from build123d import *

# Parameters (mm, degrees)
F0_W       = 355.6
F0_H       = 330.2
F0_R       = 12.7
F1_DEPTH   = 406.4
F2_DEPTH   = 73.81875
F3_SIZE    = 76.2
F4_SIZE2   = 55.4690637022
F4_SIZE    = 152.4
F4_2_SIZE2 = 55.4690637022
F4_2_SIZE  = 152.4
F5_SIZE    = 25.4
F6_SIZE2   = 76.2
F6_SIZE    = 27.7345318511


with BuildPart() as f1:
    # F0 (on Front) → F1 (new body)
    with BuildSketch(Plane.XZ):
        with Locations((-25.4, 165.1)):
            Rectangle(F0_W, F0_H)
        with Locations((-25.4, 127)):
            Circle(F0_R, mode=Mode.SUBTRACT)
        with Locations((-25.4, 127)):
            Circle(F0_R)
    extrude(amount=-F1_DEPTH)

    # F0 (on Front) → F2 (join)
    with BuildSketch(Plane.XZ):
        with Locations((-25.4, 127)):
            Circle(F0_R)
    extrude(amount=F2_DEPTH)

    # F3
    f3_edges = [f1.edges().sort_by_distance(p)[0] for p in [
        (-203.2, 203.2, 330.2),
        (152.4, 203.2, 330.2),
    ]]
    chamfer(f3_edges, length=F3_SIZE)

    # F4
    f4_edges = [f1.edges().sort_by_distance(p)[0] for p in [
        (-203.2, 203.2, 0),
    ]]
    f4_side = f1.faces().sort_by_distance((-203.2, 203.2, 127))[0]
    chamfer(f4_edges, length=F4_SIZE, length2=F4_SIZE2, reference=f4_side)

    # F4#2
    f4_2_edges = [f1.edges().sort_by_distance(p)[0] for p in [
        (152.4, 203.2, 0),
    ]]
    f4_2_side = f1.faces().sort_by_distance((152.4, 203.2, 127))[0]
    chamfer(f4_2_edges, length=F4_2_SIZE, length2=F4_2_SIZE2, reference=f4_2_side)

    # F5
    f5_edges = [f1.edges().sort_by_distance(p)[0] for p in [
        (-165.1, 0, 292.1),
        (-203.2, 0, 203.2),
        (-175.465468, 0, 76.2),
        (-25.4, 0, 0),
        (124.665468, 0, 76.2),
        (152.4, 0, 203.2),
        (114.3, 0, 292.1),
        (-25.4, 0, 330.2),
    ]]
    chamfer(f5_edges, length=F5_SIZE)

    # F6
    f6_edges = [f1.edges().sort_by_distance(p)[0] for p in [
        (-175.465468, 406.4, 76.2),
        (-203.2, 406.4, 203.2),
        (-165.1, 406.4, 292.1),
        (-25.4, 406.4, 330.2),
        (-25.4, 406.4, 0),
        (124.665468, 406.4, 76.2),
        (152.4, 406.4, 203.2),
        (114.3, 406.4, 292.1),
    ]]
    chamfer(f6_edges, length=F6_SIZE, length2=F6_SIZE2)


solid = f1.part
Check sheet for the modelled part. Datum: model origin and axes. Units: mm. A direction names the side the tool comes from. Round coordinates to 2 decimals unless told otherwise and drop trailing zeros. Loops run counter-clockwise (first coordinate to the right, second up) from the corner with the lowest first, then second, coordinate; pieces in that order, holes last. Notation, with made-up numbers: (57.25, 15.25) - (68.25, 15.25) arc R7 ccw to (68.25, 25.25) - close; hole circle Ø11 at (53, 43). An arc over 180 degrees is marked (long way). Answer as CSV lines item,"result". Start each with the question number.
Item 1: Depth check by flat-ended pin: P1, Ø8, axis at y = 4, z = 261.5, coming from the +X side; P2, Ø2, axis at y = 46, z = 96.5, coming from the -X side; P3, Ø2, axis at y = 128.5, z = 98, coming from the +X side. Enter the tip coordinate at first touch or a pass-through.
Item 2: Release check for a two-part mould opening along Y. For faces 1 (the flat face through (113.29, 12.88, 81.55)), 2 (the flat face through (124.277, 199.56, 75.133)), 3 (the flat face through (-26.822, 392.727, 291.567)) record: +Y half, -Y half, draft (parallel to the pull), parting line (faces both ways), or undercut.
Item 3: Section check A-A (x = 10). Record the boundary of the cut face in (y, z), and give its area (3 significant figures).
Item 4: Section check C-C (z = 127). Record the boundary of the cut face in (x, y), and give its area (3 significant figures).
Item 5: Scan lines: line 1 (Y direction, x = 16, z = 156); line 2 (Z direction, x = -137, y = 361.5); line 3 (Y direction, x = -123.5, z = 155.5). Record each from-to range of solid material in increasing order. Write a range as [from, to].
Item 6: Section check B-B (y = 89). Record the boundary of the cut face in (x, z), and give its area (3 significant figures).
Item 7: Section check D-D (y = -36). Record the boundary of the cut face in (x, z).
Item 8: Set-up check for faces 4 (the cylindrical face through (-28.15, -36.39, 114.6)), 5 (the flat face through (-175.077, 199.56, 75.133)): record each of +Z, -Z, +X, -X, +Y, -Y from which the full face is reachable in a straight line by a thin tool's end or side.
Report:
1,P1,"stops at x = 121.56"
1,P2,"stops at x = -183.22"
1,P3,"stops at x = 132.96"
2,face 1,"-Y half"
2,face 2,"draft"
2,face 3,"+Y half"
3,outline,"(0, 25.4) - (25.4, 0) - (378.67, 0) - (406.4, 76.2) - (406.4, 254) - (378.67, 330.2) - (25.4, 330.2) - (0, 304.8) - close"
3,area,"131,000 mm2"
4,outline,"(-193.96, 25.4) - (-166.93, 0) - (-38.1, 0) - (-38.1, -73.82) - (-12.7, -73.82) - (-12.7, 0) - (116.13, 0) - (143.16, 25.4) - (143.16, 378.67) - (62.06, 406.4) - (-112.86, 406.4) - (-193.96, 378.67) - close"
4,area,"136,000 mm2"
5,line 1,"y = [0, 406.4]"
5,line 2,"z = [0, 320.2]"
5,line 3,"y = [0, 406.31]"
6,outline,"(-203.2, 152.4) - (-147.73, 0) - (96.93, 0) - (152.4, 152.4) - (152.4, 254) - (76.2, 330.2) - (-127, 330.2) - (-203.2, 254) - close"
6,area,"103,000 mm2"
7,outline,"circle Ø25.4 at (-25.4, 127)"
8,face 4,"-Y"
8,face 5,"-Z, -X, +Y, -Y"
